from build123d import *

# Parameters (mm, degrees)
F0_R          = 3.302
F0_R_2        = 15.875
F1_DEPTH      = 9.525
F0_R_3        = 13.335
F2_DEPTH      = 2.54
F5_DEPTH      = 8.636
F6_T1_DEPTH   = 2.3368
F6_T3_DEPTH   = 2.3368
F6_T5_DEPTH   = 2.3368
F3_R          = 6.35
F3_R_2        = 3.302
F7_DEPTH      = 6.35
F11_R         = 1.5875
F12_DEPTH     = 6.35
F9_R          = 1.5875
F13_DEPTH     = 6.35
F10_R         = 1.5875
F14_DEPTH     = 8.382
F16_DEPTH     = 5.6642
F15_W         = 15.0114
F15_H         = 10.748598603
F17_DEPTH     = 2.8448
F18_T4_DEPTH  = 29.6432475283
F18_T9_DEPTH  = 29.6432475283
F18_T14_DEPTH = 29.6432475283
F18_T19_DEPTH = 29.6432475283
F19_W         = 11.2522
F19_H         = 5.9944
F20_DEPTH     = 13.9954
F21_T1_DEPTH  = 20.5629100612
F22_T1_DEPTH  = 20.5167471751
F23_R         = 3.5052
F24_R         = 3.5052
F25_DEPTH     = 7.62


# Not quite as in the source:
# - a fillet or chamfer that OpenCascade refuses, or shapes differently, is made with other operations: its cross-section is extruded or revolved along the edge and cut away or added
# - a feature names something its author has since deleted; it is built from what else it names


with BuildPart() as f1:
    # F0 (on Top) → F1 (new body)
    with BuildSketch(Plane.XY):
        with BuildLine():
            Line((39.3578503288, 46.2881387371), (6.9933568382, 57.0169901512))
            ThreePointArc((6.9933568382, 57.0169901512), (0, 58.145934), (-6.9933568382, 57.0169901512))
            Line((-6.9933568382, 57.0169901512), (-39.3578503288, 46.2881387371))
            ThreePointArc((-39.3578503288, 46.2881387371), (-46.548869386, 38.4390523526), (-43.6441157783, 28.1978942818))
            Line((-43.6441157783, 28.1978942818), (-32.9057, 17.459532603))
            Line((-32.9057, 17.459532603), (-32.9057, -8.529066))
            Line((-32.9057, -8.529066), (-17.8943, -8.529066))
            Line((-17.8943, -8.529066), (-17.8943, 2.4482082294))
            Line((-17.8943, 2.4482082294), (-7.72300081, -7.7230397182))
            ThreePointArc((-7.72300081, -7.7230397182), (0, -10.922), (7.72300081, -7.7230397182))
            Line((7.72300081, -7.7230397182), (17.8943, 2.4482082294))
            Line((17.8943, 2.4482082294), (17.8943, -8.529066))
            Line((17.8943, -8.529066), (32.9057, -8.529066))
            Line((32.9057, -8.529066), (32.9057, 17.459532603))
            Line((32.9057, 17.459532603), (43.6441157783, 28.1978942818))
            ThreePointArc((43.6441157783, 28.1978942818), (46.548869386, 38.4390523526), (39.3578503288, 46.2881387371))
        make_face()
        Circle(F0_R, mode=Mode.SUBTRACT)
        with Locations((-35.9211149683, 35.920934)):
            Circle(F0_R, mode=Mode.SUBTRACT)
        with Locations((0, 35.920934)):
            Circle(F0_R_2, mode=Mode.SUBTRACT)
        with Locations((35.9211149683, 35.920934)):
            Circle(F0_R, mode=Mode.SUBTRACT)
    extrude(amount=F1_DEPTH)

    # F0 (on Top) → F2 (join)
    with BuildSketch(Plane.XY):
        with Locations((0, 35.920934)):
            Circle(F0_R_2)
        with Locations((0, 35.920934)):
            Circle(F0_R_3, mode=Mode.SUBTRACT)
    extrude(amount=F2_DEPTH)

    # F4 (on face) → F5 (cut)
    with BuildSketch(Plane.XY.offset(9.525)):
        Polygon((-42.2711149683, 32.695134), (-42.2711149683, 35.920934), (-42.2711149683, 39.146734), (-44.6079149683, 39.146734), (-44.6079149683, 32.695134), align=None)
        Polygon((42.2711149683, 39.146734), (42.2711149683, 35.920934), (42.2711149683, 32.695134), (44.6079149683, 32.695134), (44.6079149683, 39.146734), align=None)
        Polygon((3.2258, -6.35), (0, -6.35), (-3.2258, -6.35), (-3.2258, -8.6868), (3.2258, -8.6868), align=None)
    extrude(amount=-F5_DEPTH, mode=Mode.SUBTRACT)

    # F6: chamfer of 3.175 x 5.499261314 on 6 edges, made by hand

    # F6_s2 → F6_t1 (join)
    with BuildSketch(Plane.YZ.offset(-44.6079149683)):
        Polygon((39.146734, 4.064), (33.647472686, 0.889), (39.146734, 0.889), align=None)
        Polygon((32.695134, 4.064), (38.194395314, 0.889), (32.695134, 0.889), align=None)
    extrude(amount=F6_T1_DEPTH)

    # F6_s4 → F6_t3 (join)
    with BuildSketch(Plane.XZ.offset(6.35)):
        Polygon((3.2258, 4.064), (-2.273461314, 0.889), (3.2258, 0.889), align=None)
        Polygon((-3.2258, 4.064), (2.273461314, 0.889), (-3.2258, 0.889), align=None)
    extrude(amount=F6_T3_DEPTH)

    # F6_s6 → F6_t5 (join)
    with BuildSketch(Plane.YZ.offset(42.2711149683)):
        Polygon((39.146734, 4.064), (33.647472686, 0.889), (39.146734, 0.889), align=None)
        Polygon((32.695134, 4.064), (38.194395314, 0.889), (32.695134, 0.889), align=None)
    extrude(amount=F6_T5_DEPTH)

    # F3 (on face) → F7 (join)
    with BuildSketch(Plane.XY.offset(9.525)):
        with Locations((-35.9211149683, 35.920934)):
            Circle(F3_R)
        with Locations((-35.9211149683, 35.920934)):
            Circle(F3_R_2, mode=Mode.SUBTRACT)
        Circle(F3_R)
        Circle(F3_R_2, mode=Mode.SUBTRACT)
        with Locations((35.9211149683, 35.920934)):
            Circle(F3_R)
        with Locations((35.9211149683, 35.920934)):
            Circle(F3_R_2, mode=Mode.SUBTRACT)
    extrude(amount=F7_DEPTH)

    # F8: fillet of radius 6.096 on 3 edges, made by hand

    # F8_s1 → F8_t2 (revolve, cut)
    with BuildSketch(Plane.XZ.offset(-35.920934)):
        with BuildLine():
            ThreePointArc((-29.5711149683, 10.5957091385), (-30.3878241069, 13.6437091385), (-32.6191149683, 15.875))
            Line((-32.6191149683, 15.875), (-29.5711149683, 15.875))
            Line((-29.5711149683, 15.875), (-29.5711149683, 10.5957091385))
        make_face()
    revolve(axis=Axis((-35.9211149683, 35.920934, 15.875), (0, 0, 1)), mode=Mode.SUBTRACT)

    # F8_s3 → F8_t4 (revolve, cut)
    with BuildSketch(Plane.XZ.offset(-35.920934)):
        with BuildLine():
            ThreePointArc((42.2711149683, 10.5957091385), (41.4544058298, 13.6437091385), (39.2231149683, 15.875))
            Line((39.2231149683, 15.875), (42.2711149683, 15.875))
            Line((42.2711149683, 15.875), (42.2711149683, 10.5957091385))
        make_face()
    revolve(axis=Axis((35.9211149683, 35.920934, 15.875), (0, 0, 1)), mode=Mode.SUBTRACT)

    # F8_s5 → F8_t6 (revolve, cut)
    with BuildSketch(Plane.XZ):
        with BuildLine():
            ThreePointArc((6.35, 10.5957091385), (5.5332908615, 13.6437091385), (3.302, 15.875))
            Line((3.302, 15.875), (6.35, 15.875))
            Line((6.35, 15.875), (6.35, 10.5957091385))
        make_face()
    revolve(axis=Axis((0, 0, 15.875), (0, 0, 1)), mode=Mode.SUBTRACT)

    # F11 (on face) → F12 (cut, symmetric)
    with BuildSketch(Plane(origin=(44.6079149683, 0, 0), x_dir=(0, -1, 0), z_dir=(-1, 0, 0))):
        with Locations((-35.8627085169, 5.8928)):
            Circle(F11_R)
    extrude(amount=F12_DEPTH, both=True, mode=Mode.SUBTRACT)

    # F9 (on face) → F13 (cut, symmetric)
    with BuildSketch(Plane.YZ.offset(-44.6079149683)):
        with Locations((35.8627085169, 5.8928)):
            Circle(F9_R)
    extrude(amount=F13_DEPTH, both=True, mode=Mode.SUBTRACT)

    # F10 (on face) → F14 (cut, symmetric)
    with BuildSketch(Plane(origin=(0, -8.6868, 0), x_dir=(-1, 0, 0), z_dir=(0, 1, 0))):
        with Locations((0.0582254831, 5.8928)):
            Circle(F10_R)
    extrude(amount=F14_DEPTH, both=True, mode=Mode.SUBTRACT)

    # F15 (on face) → F16 (join)
    with BuildSketch(Plane.XY.offset(9.525)):
        Polygon((17.8943, 6.710934), (17.8943, 2.4482082294), (17.8943, -8.529066), (32.9057, -8.529066), (32.9057, 6.710934), align=None)
        Polygon((-32.9057, -8.529066), (-17.8943, -8.529066), (-17.8943, 2.4482082294), (-17.8943, 6.710934), (-32.9057, 6.710934), align=None)
    extrude(amount=F16_DEPTH)

    # F15 (on face) → F17 (join)
    with BuildSketch(Plane.XY.offset(9.525)):
        with Locations((-25.4, 12.0852333015)):
            Rectangle(F15_W, F15_H)
        with Locations((25.4, 12.0852333015)):
            Rectangle(F15_W, F15_H)
    extrude(amount=F17_DEPTH)

    # F18: chamfer of 2.8448 on 4 edges, made by hand


with BuildPart() as f18_tool2:
    # F18_s3 → F18_t4 (new body)
    with BuildSketch(Plane.YZ.offset(-10.5783762358)):
        Polygon((14.614732603, 12.3698), (17.459532603, 9.525), (17.459532603, 12.3698), align=None)
    extrude(amount=-F18_T4_DEPTH)

    split(bisect_by=Plane.XY.offset(9.525), keep=Keep.TOP)


with BuildPart() as f1_1:
    add(f1.part)

    # F18_t1: cut F18_tool2
    add(f18_tool2.part, mode=Mode.SUBTRACT)


with BuildPart() as f18_tool7:
    # F18_s8 → F18_t9 (new body)
    with BuildSketch(Plane.YZ.offset(40.2216237642)):
        Polygon((17.459532603, 9.525), (14.614732603, 12.3698), (17.459532603, 12.3698), align=None)
    extrude(amount=-F18_T9_DEPTH)

    split(bisect_by=Plane.XY.offset(9.525), keep=Keep.TOP)


with BuildPart() as f1_2:
    add(f1_1.part)

    # F18_t6: cut F18_tool7
    add(f18_tool7.part, mode=Mode.SUBTRACT)


with BuildPart() as f18_tool12:
    # F18_s13 → F18_t14 (new body)
    with BuildSketch(Plane.YZ.offset(-10.5783762358)):
        Polygon((6.710934, 12.3444), (3.866134, 15.1892), (6.710934, 15.1892), align=None)
    extrude(amount=-F18_T14_DEPTH)

    split(bisect_by=Plane.XY.offset(12.3698), keep=Keep.TOP)


with BuildPart() as f1_3:
    add(f1_2.part)

    # F18_t11: cut F18_tool12
    add(f18_tool12.part, mode=Mode.SUBTRACT)


with BuildPart() as f18_tool17:
    # F18_s18 → F18_t19 (new body)
    with BuildSketch(Plane.YZ.offset(40.2216237642)):
        Polygon((6.710934, 12.3444), (3.866134, 15.1892), (6.710934, 15.1892), align=None)
    extrude(amount=-F18_T19_DEPTH)

    split(bisect_by=Plane.XY.offset(12.3698), keep=Keep.TOP)


with BuildPart() as f1_4:
    add(f1_3.part)

    # F18_t16: cut F18_tool17
    add(f18_tool17.part, mode=Mode.SUBTRACT)

    # F19 (on face) → F20 (cut)
    with BuildSketch(Plane.XY.offset(15.1892)):
        with Locations((-25.4, -3.042666)):
            Rectangle(F19_W, F19_H)
        with Locations((25.4, -3.042666)):
            Rectangle(F19_W, F19_H)
    extrude(amount=-F20_DEPTH, mode=Mode.SUBTRACT)

    # F21: chamfer of 3.2512 x 5.6312435856 on 3 edges, made by hand

    # F21_s2 → F21_t1 (join)
    with BuildSketch(Plane.XZ.offset(-14.5230440612)):
        Polygon((-19.7739, 4.445), (-25.4051435856, 1.1938), (-19.7739, 1.1938), align=None)
        Polygon((-31.0261, 4.445), (-25.3948564144, 1.1938), (-31.0261, 1.1938), align=None)
        Polygon((31.0261, 4.445), (25.3948564144, 1.1938), (31.0261, 1.1938), align=None)
    extrude(amount=F21_T1_DEPTH)

    # F22: chamfer of 5.6134 x 3.2408980011 on 1 edges, made by hand

    # F22_s2 → F22_t1 (join)
    with BuildSketch(Plane.XZ.offset(-14.4768811751)):
        Polygon((19.7739, 4.4346980011), (25.3873, 1.1938), (19.7739, 1.1938), align=None)
    extrude(amount=F22_T1_DEPTH)

    # F23 (on face) + F24 (on face) → F25 (cut, symmetric)
    with BuildSketch(Plane(origin=(0, -6.039866, 0), x_dir=(-1, 0, 0), z_dir=(0, 1, 0))):
        with Locations((25.4, 7.6932303495)):
            Circle(F23_R)
    with BuildSketch(Plane(origin=(0, -6.039866, 0), x_dir=(-1, 0, 0), z_dir=(0, 1, 0))):
        with Locations((-25.3948564144, 7.6962)):
            Circle(F24_R)
    extrude(amount=F25_DEPTH, both=True, mode=Mode.SUBTRACT)


solid = f1_4.part
Build history of the part. All positions in model axes, mm. A direction names the side the tool comes from. Round coordinates to 2 decimals unless told otherwise and drop trailing zeros. Write each loop counter-clockwise with the first axis right and the second up, starting at its lowest first coordinate (ties: lowest second). Pieces come first, ordered by that corner, then holes. Notation, with made-up numbers: M 74.5,88 L 107.5,88 A15 ccw 107.5,109 Z; hole C -16,58 d3. An arc over 180 degrees is marked long. Answer as a JSON object with one key per item and string values. Group by question number.
(1) Cut at A-A (y = 44.5). Give the cut face in (x, z) (3 decimals).
(2) Mould opens along Z. For faces 5 (the flat face through (1.64, -7.5, 3.15)), 6 (the cylindrical face through (-21.9, 0.76, 7.85)), 7 (the flat face through (-12.88, -2.566, 4.696)) say: pulls with the +Z half, pulls with the -Z half, needs draft (parallel to the pull), parting line crosses it, or undercut.
(3) Drill centre lines: L1, parallel to Y at x = 2.5, z = 2; L2, parallel to X at y = -6.5, z = 1; L3, parallel to Z at x = -25.4, y = -7.05. Where is each one in solid material? Low to high.
(4) Which spindle directions (+Z, -Z, +X, -X, +Y, -Y) get a long thin tool onto all of the face, cutting with end or side? Do faces 1 (the flat face through (-1.64, -7.5, 3.15)), 2 (the flat face through (12.737, -2.709, 4.696)), 3 (the flat face through (17.894, -1, 7)), 4 (the cylindrical face through (45.7, 37.1, 4.9)). Say none if no direction does.
(5) Flat gauge pins, fed straight in: pin 1 (3 mm diameter, centred on y = 35, z = 6, fed in from -X); pin 2 (5 mm diameter, centred on y = 14, z = 8.5, fed in from +X); pin 3 (1.9 mm diameter, centred on y = 35.86, z = 5.89, fed in from +X); pin 4 (1 mm diameter, centred on x = 14, z = 11, fed in from -Y). Where does each tip first touch, or does it go through?
(6) Cut at C-C (z = 14). Give the number of separate pieces and of enclosed holes in the cut face, and give its area (3 significant figures).
(7) Cut at B-B (x = 12). Give the cut face in (y, z) (3 decimals).
Responses:
{
 "1": {"outline": "M -42.681,0 L -10.209,0 L -10.209,2.54 L -13.357,2.54 L -13.357,9.525 L -42.681,9.525 Z; M 10.209,0 L 42.681,0 L 42.681,9.525 L 13.357,9.525 L 13.357,2.54 L 10.209,2.54 Z"},
 "2": {"face 5": "pulls with the +Z half", "face 6": "undercut", "face 7": "needs draft"},
 "3": {"L1": "y = -10.63 to -2.16, 2.16 to 22.82, 49.02 to 58", "L2": "x = -32.91 to -17.89, -8.95 to 8.95, 17.89 to 32.91", "L3": "z = 0 to 4.19, 11.2 to 15.19"},
 "4": {"face 1": "+Z", "face 2": "+Z, -Z, -Y", "face 3": "+Z, -Y", "face 4": "+X"},
 "5": {"pin 1": "stops at x = -46.83", "pin 2": "stops at x = 32.91", "pin 3": "stops at x = 32.78", "pin 4": "passes through"},
 "6": {"separate pieces": "5", "enclosed holes": "5", "area": "436 mm2"},
 "7": {"outline": "M -3.446,0 L 30.105,0 L 30.105,2.54 L 25.528,2.54 L 25.528,9.525 L -3.446,9.525 Z; M 41.737,0 L 55.357,0 L 55.357,9.525 L 46.314,9.525 L 46.314,2.54 L 41.737,2.54 Z"}
}
